```python
from build123d import *

# Parameters (mm, degrees)
SKETCH1_R                = 8.7
BASE_EXTRUDE_DEPTH       = 25.2
BASE_EXTRUDE_DEPTH_BACK  = 25.2
SKETCH2_R                = 8
STROKECHAMBER_DEPTH      = 15.2
STROKECHAMBER_DEPTH_BACK = 15.2
CHAMFER1_SIZE            = 0.5
SKETCH3_R                = 2.55
THRUBORE_DEPTH           = 26.2
SKETCH4_R                = 2.55
CUT_EXTRUDE1_DEPTH       = 51.4


with BuildPart() as part:
    # Sketch1 → Base-Extrude (new body, two sides)
    with BuildSketch(Plane.XY) as base_extrude_sk:
        Circle(SKETCH1_R)
    extrude(amount=BASE_EXTRUDE_DEPTH)
    extrude(base_extrude_sk.sketch, amount=-BASE_EXTRUDE_DEPTH_BACK)

    # Sketch2 → StrokeChamber (cut, two sides)
    with BuildSketch(Plane.XY) as strokechamber_sk:
        Circle(SKETCH2_R)
    extrude(amount=STROKECHAMBER_DEPTH, mode=Mode.SUBTRACT)
    extrude(strokechamber_sk.sketch, amount=-STROKECHAMBER_DEPTH_BACK, mode=Mode.SUBTRACT)

    # Chamfer1
    chamfer1_edges = [part.edges().sort_by_distance(p)[0] for p in [
        (-8.7, 0, 25.2),
        (-8.7, 0, -25.2),
    ]]
    chamfer(chamfer1_edges, length=CHAMFER1_SIZE)

    # Sketch3 → Thrubore (cut, through all)
    with BuildSketch(Plane.XY):
        Circle(SKETCH3_R)
    extrude(amount=THRUBORE_DEPTH, mode=Mode.SUBTRACT)

    # Sketch4 → Cut-Extrude1 (cut, through all)
    with BuildSketch(Plane.XY.offset(25.2)):
        Circle(SKETCH4_R)
    extrude(amount=-CUT_EXTRUDE1_DEPTH, mode=Mode.SUBTRACT)


solid = part.part
```
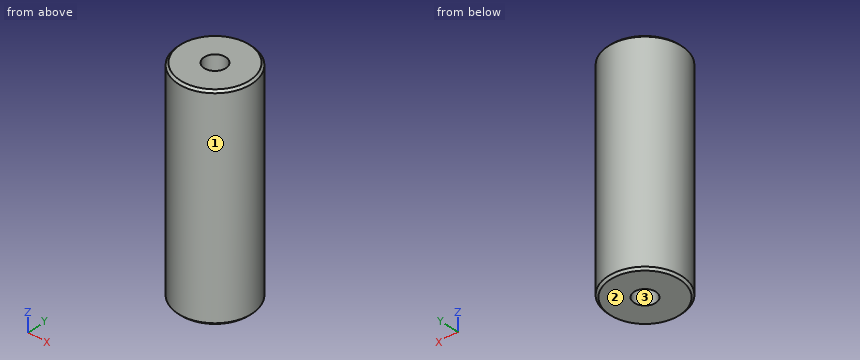
Verification items for the finished model (mm, model axes). Face numbers are marked on the shaded views. Round coordinates to 2 decimals unless told otherwise and drop trailing zeros. Order: outer loops, then holes, each group sorted by start corner. A loop starts at its lowest first (then second) coordinate and runs counter-clockwise, first axis right, second up. Notation, with made-up numbers: (26.25, 84) - (33.25, 84) arc R22 ccw to (33.25, 120) - close; hole circle Ø10 at (1, 46). An arc over 180 degrees is marked (long way). Use CSV: the item, a comma, the result in double quotes.
(1) Section check D-D on z = 17. Record the boundary of the cut face in (x, y), and give its area (3 significant figures).
Entries:
outline,"circle Ø17.4 at (0, 0); hole circle Ø5.1 at (0, 0)"
area,"217 mm^2"
(2) Gauge pin test, flat ends, axial feed: pin 1 Ø3 at (x, z) = (6, 17.5) entering from +Y; pin 2 Ø3 at (y, z) = (-6.5, -13) entering from +X; pin 3 Ø1 at (x, z) = (5, 16) entering from -Y. Record the tip position at first contact, or that the pin passes through.
Entries:
pin 1,"y = 7.45"
pin 2,"x = 7.12"
pin 3,"y = -7.45"
(3) Thickness scan on probe 1 along Z at (x, y) = (2.25, 2); probe 2 along Y at (x, z) = (0, -19.25); probe 3 along Y at (x, z) = (0, 7.5). Record the ranges inside material, lowest first. Write a range as from..to.
Entries:
probe 1,"-25.2..-15.2, 15.2..25.2"
probe 2,"-8.7..-2.55, 2.55..8.7"
probe 3,"-8.7..-8, 8..8.7"
(4) Mould release check, pull along Y, two halves, no side actions. Record for the marked faces 1, 2 and 3: released by +Y, released by -Y, zero draft, split by the parting line, or undercut.
Entries:
face 1,"split by the parting line"
face 2,"zero draft"
face 3,"undercut"
(5) Section check A-A on y = 0. Record the boundary of the cut face in (x, z), and give its area (3 significant figures).
Entries:
outline,"(-8.7, -24.7) - (-8.2, -25.2) - (-2.55, -25.2) - (-2.55, -15.2) - (-8, -15.2) - (-8, 15.2) - (-2.55, 15.2) - (-2.55, 25.2) - (-8.2, 25.2) - (-8.7, 24.7) - close; (2.55, -25.2) - (8.2, -25.2) - (8.7, -24.7) - (8.7, 24.7) - (8.2, 25.2) - (2.55, 25.2) - (2.55, 15.2) - (8, 15.2) - (8, -15.2) - (2.55, -15.2) - close"
area,"288 mm^2"
(6) Section check C-C on z = -3.5. Record the boundary of the cut face in (x, y).
Entries:
outline,"circle Ø17.4 at (0, 0); hole circle Ø16 at (0, 0)"
